from build123d import *

# Parameters (mm, degrees)
SKETCH1_R           = 1.6
BOSS_EXTRUDE2_DEPTH = 2


with BuildPart() as part:
    # Sketch1 → Boss-Extrude2 (new body)
    with BuildSketch(Plane.XY):
        with BuildLine():
            Line((0, -3), (9.999997972, -3))
            ThreePointArc((9.999997972, -3), (12.496148784, -1.664100694), (12.769228838, 1.15384592))
            Line((12.769228838, 1.15384592), (9.189348108, 9.745561719))
            ThreePointArc((9.189348108, 9.745561719), (4.999998986, 12.538461389), (0.810649864, 9.745561719))
            Line((0.810649864, 9.745561719), (-2.769230867, 1.15384592))
            ThreePointArc((-2.769230867, 1.15384592), (-2.496150813, -1.664100694), (0, -3))
        make_face()
        with Locations((9.999997972, 0)):
            Circle(SKETCH1_R, mode=Mode.SUBTRACT)
        Circle(SKETCH1_R, mode=Mode.SUBTRACT)
        with Locations((4.999998986, 8)):
            Circle(SKETCH1_R, mode=Mode.SUBTRACT)
    extrude(amount=BOSS_EXTRUDE2_DEPTH)


solid = part.part
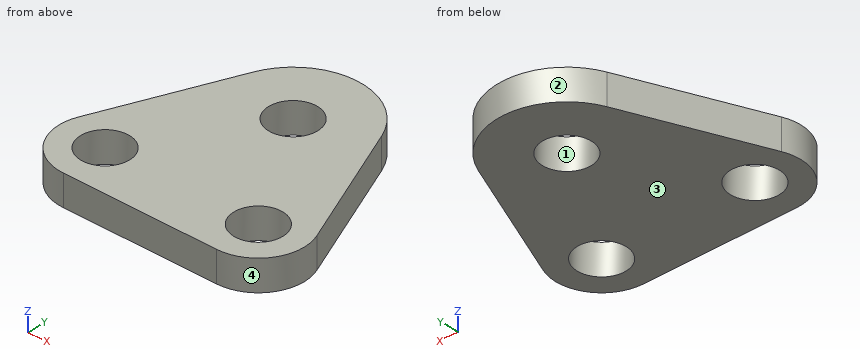
For this review, take the finished solid that the model builds, in its own axes (mm). Face numbers are marked on the shaded views. Give positions to 0.01 mm unless a question says otherwise; leave off trailing zeros. Loops run counter-clockwise (first coordinate to the right, second up) from the corner with the lowest first, then second, coordinate; pieces in that order, holes last. Notation, with made-up numbers: M -13,73 L 28,73 A24 ccw 28,95 Z; hole C -17,66.25 d10. An arc over 180 degrees is marked long. Put each result on its own line as item: value. Start each with the question number.
(1) Wall thickness on L1, parallel to Y at x = -1.25, z = 1.95; L2, parallel to Y at x = 4.5, z = 0.2; L3, parallel to X at y = 1.25, z = 1.55: over which ranges is each line inside the solid? List them lowest first.
(2) Add section A-A, the plane x = 5. Write out the cut boundary in (y, z), then the cut area to 3 significant figures.
(3) For pin 1 (1 mm diameter, centred on x = 6, z = 1, fed in from +Y); pin 2 (8 mm diameter, centred on x = 0, y = 2, fed in from -Z), all flat-tipped, find the tip position at first contact; note any pin that passes through.
(4) Add section B-B, the plane z = 0.25. Write out the cut boundary in (x, y).
(5) Add section D-D, the plane x = 7.25. Write out the cut boundary in (y, z), then the cut area to 3 significant figures.
(6) Add section C-C, the plane y = 9. Write out the cut boundary in (x, z), then the cut area to 3 significant figures.
(7) The part is to be moulded in two halves that separate along Y. For the marked faces 1, 2, 3 and 4, say which applies: +Y half, -Y half, draft (parallel to the pull), parting line (faces both ways), or undercut.
Result:
1. L1: y = -2.73 to -1, 1 to 4.8
1. L2: y = -3 to 6.48, 9.52 to 12.51
1. L3: x = -2.73 to -1, 1 to 9, 11 to 12.73
2. outline: M -3,0 L 6.4,0 L 6.4,2 L -3,2 Z; M 9.6,0 L 12.54,0 L 12.54,2 L 9.6,2 Z
2. area: 24.7 mm^2
3. pin 1: stops at y = 12.51
3. pin 2: stops at z = 0
4. outline: M -2.77,1.15 A3 ccw 0,-3 L 10,-3 A3 ccw 12.77,1.15 L 9.19,9.75 A4.54 ccw 0.81,9.75 Z; hole C 0,0 d3.2; hole C 5,8 d3.2; hole C 10,0 d3.2
5. outline: M -3,0 L 11.94,0 L 11.94,2 L -3,2 Z
5. area: 29.9 mm^2
6. outline: M 0.5,0 L 3.75,0 L 3.75,2 L 0.5,2 Z; M 6.25,0 L 9.5,0 L 9.5,2 L 6.25,2 Z
6. area: 13.0 mm^2
7. face 1: undercut
7. face 2: +Y half
7. face 3: draft
7. face 4: parting line
